from build123d import *

# Parameters (mm, degrees)
F0_W     = 50.8
F0_H     = 50.8
F1_DEPTH = 12.7
F2_W     = 51.009607
F2_H     = 12.687672
F3_DEPTH = 38.1
F4_R     = 9.780589
F5_DEPTH = 12.7


with BuildPart() as f1:
    # F0 (on Front) → F1 (new body)
    with BuildSketch(Plane.XZ):
        with Locations((25.4, 25.4)):
            Rectangle(F0_W, F0_H)
    extrude(amount=F1_DEPTH)

    # F2 (on Front) → F3 (join)
    with BuildSketch(Plane.XZ):
        with Locations((25.504803, 44.665778)):
            Rectangle(F2_W, F2_H)
    extrude(amount=F3_DEPTH)

    # F4 (on face) → F5 (cut, through all)
    with BuildSketch(Plane.XZ.offset(12.7)):
        with Locations((24.682367, 17.329346)):
            Circle(F4_R)
    extrude(amount=-F5_DEPTH, mode=Mode.SUBTRACT)


solid = f1.part
Design review of the part built by this model. Coordinates are the model's own, in mm. A direction names the side the tool comes from. Round coordinates to 2 decimals unless told otherwise and drop trailing zeros. Order: outer loops, then holes, each group sorted by start corner. A loop starts at its lowest first (then second) coordinate and runs counter-clockwise, first axis right, second up. Notation, with made-up numbers: M 78,21 L 101,21 A21 cw 101,43 Z; hole C -40,2.25 d7. An arc over 180 degrees is marked long. Answer as CSV lines item,"result". Start each with the question number.
1) Add section D-D (x = 38.5). Give the boundary of the cut face in (y, z).
2) For pin 1 Ø8 at (x, z) = (19, 8.5) entering from -Y; pin 2 Ø5 at (x, y) = (12, -19) entering from -Z; pin 3 Ø1 at (x, z) = (35.5, 29.5) entering from +Y; pin 4 Ø10 at (y, z) = (-7, 20) entering from +X, all flat-tipped, find the tip position at first contact; note any pin that passes through.
3) Wall thickness on line 1 along X through (y, z) = (-8.5, 7.5); line 2 along Z through (x, y) = (4, -26.5); line 3 along Y through (x, z) = (41, 29): over which ranges is each line inside the solid? List them lowest first. Write a range as [from, to].
4) Tool access review of faces 5 (the face through (25, -12.7, 28)), 6 (the face through (25, -19, 51.01)): name each direction out of +Z, -Z, +X, -X, +Y, -Y from which nothing blocks a thin tool from reaching the whole face with its end or side.
5) Add section C-C (y = -11). Give the boundary of the cut face in (x, z), then the cut area to 3 significant figures.
6) Add section A-A (z = 9.5). Give the boundary of the cut face in (x, y), then the cut area to 3 significant figures.
7) Add section B-B (x = 29.5). Give the boundary of the cut face in (y, z).
8) The part is to be moulded in two halves that separate along X. For faces 1 (the face through (25, 0, 32)), 2 (the face through (0, -6, 19)), 3 (the face through (14.91, -6.44, 17.76)), 4 (the face through (50.8, -6, 19)), say which applies: +X half, -X half, draft (parallel to the pull), parting line (faces both ways), or undercut.
Resolved:
1,outline,"M -38.1,38.32 L -12.7,38.32 L -12.7,0 L 0,0 L 0,51.01 L -38.1,51.01 Z"
2,pin 1,"y = -12.7"
2,pin 2,"z = 38.32"
2,pin 3,"y = 0"
2,pin 4,"x = 50.8"
3,line 1,"[0, 50.8]"
3,line 2,"[38.32, 51.01]"
3,line 3,"[-12.7, 0]"
4,face 5,"-Z, +X, -X, -Y"
4,face 6,"+Z, +X, -X, +Y, -Y"
5,outline,"M 0,0 L 50.8,0 L 50.8,38.32 L 51.01,38.32 L 51.01,51.01 L 0,51.01 Z; hole C 24.68,17.33 d19.56"
5,area,"2,290 mm^2"
6,outline,"M 0,-12.7 L 18.82,-12.7 L 18.82,0 L 0,0 Z; M 30.54,-12.7 L 50.8,-12.7 L 50.8,0 L 30.54,0 Z"
6,area,"496 mm^2"
7,outline,"M -38.1,38.32 L -12.7,38.32 L -12.7,25.84 L 0,25.84 L 0,51.01 L -38.1,51.01 Z; M -12.7,0 L 0,0 L 0,8.82 L -12.7,8.82 Z"
8,face 1,"draft"
8,face 2,"-X half"
8,face 3,"undercut"
8,face 4,"+X half"
